Autodesk Inventor part; units mm, degrees
ref_plane "YZ Plane" through (0, 0, 0) normal (1, 0, 0) x (0, 1, 0)
ref_plane "XZ Plane" through (0, 0, 0) normal (0, 1, 0) x (-1, 0, 0)
ref_plane "XY Plane" through (0, 0, 0) normal (0, 0, 1) x (1, 0, 0)
sketch "Sketch1" plane through (0, 0, 0) normal (0, 1, 0) x (-1, 0, 0)
  line L0 (0, 0) -> (12.5, 0)
  line L1 (12.5, 0) -> (12.5, -22.9)
  line L2 (12.5, -22.9) -> (0, -22.9)
  line L3 (0, -22.9) -> (0, 0)
  line L4 (12.5, 0) -> (13, 0)
  line L5 (0, -22.9) -> (-0.5, -22.9)
  line L6 (13, 0) -> (13, 4.65)
  line L7 (-0.5, -22.9) -> (-0.5, -27.55)
  line L8 (13, 4.65) -> (-0.5, 4.65)
  line L9 (-0.5, 4.65) -> (-0.5, -27.55)
  line L10 (-0.5, -27.55) -> (13, -27.55)
  line L11 (13, -27.55) -> (13, 4.65)
  line L12 (6.25, 0) -> (6.25, 2.45)
  line L13 (6.25, -22.9) -> (6.25, -25.35)
  circle A0 centre (6.25, 2.45) radius 0.75
  circle A1 centre (6.25, -25.35) radius 0.75
  dimension "d0" = 12.5
  dimension "d1" = 22.9
  dimension "d2" = 0.5
  dimension "d3" = 0.5
  dimension "d4" = 4.65
  dimension "d5" = 4.65
  dimension "d6" = 2.45
  dimension "d7" = 2.45
  dimension "d8" = 1.5
  dimension "d9" = 1.5
extrude "Extrusion1" add sketch "Sketch1" along normal blind 17.3 contours A0 | L3 L5 L9 L8 L6 L4 L0 | A1 | L2 L1 L4 L11 L10 L7 L5
extrude "Extrusion2" add sketch "Sketch1" against normal blind 1 contours A0 | L3 L5 L9 L8 L6 L4 L0 | L0 L1 L2 L3 | A1 | L2 L1 L4 L11 L10 L7 L5
sketch "Sketch2" plane through (0, -1, 0) normal (0, -1, 0) x (1, 0, 0)
  line L0 (0.5, 4.65) -> (0.5, -27.55)
  line L1 (-12.5, -22.9) -> (0, -22.9)
  line L2 (-13, -27.55) -> (-13, 4.65)
  line L3 (-13, 4.65) -> (-13, 0)
  line L4 (-13, 0) -> (-6.3, 0)
  line L5 (0, 0) -> (-12.5, 0)
  line L6 (-6.3, 0) -> (-6.3, -5.6)
  circle A0 centre (-6.3, -5.6) radius 3.025
  dimension "d20" = 4.65
  dimension "d21" = 6.7
  dimension "d22" = 5.6
  dimension "d23" = 6.05
extrude "Extrusion3" add sketch "Sketch2" along normal blind 4.7
sketch "Sketch3" plane through (-6.3, -5.7, -5.6) normal (0, -1, 0) x (1, 0, 0)
  line L0 (0, 0) -> (1.385, 0)
  line L1 (0, 0) -> (0, 1.385)
  line L2 (1.385, 0) -> (1.385, 0.32)
  line L3 (0, 1.385) -> (-0.32, 1.385)
  line L4 (-0.32, 1.385) -> (0.32, 1.385)
  line L5 (0.32, 1.385) -> (0.32, -1.385)
  line L6 (0.32, -1.385) -> (-0.32, -1.385)
  line L7 (-0.32, -1.385) -> (-0.32, 1.385)
  line L8 (1.385, 0.32) -> (-1.385, 0.32)
  line L9 (-1.385, 0.32) -> (-1.385, -0.32)
  line L10 (-1.385, -0.32) -> (1.385, -0.32)
  line L11 (1.385, -0.32) -> (1.385, 0.32)
  point P0 (6.3, 5.6)
  point P1 (-0.32, 0.32)
  point P2 (-0.32, -0.32)
  point P3 (0.32, -0.32)
  point P4 (0.32, 0.32)
  dimension "d24" = 1.385
  dimension "d25" = 1.385
  dimension "d26" = 0.32
  dimension "d27" = 0.32
  dimension "d28" = 0.64
  dimension "d30" = 2.77
  dimension "d31" = 0.64
  dimension "d32" = 2.77
extrude "Extrusion4" [suppressed]
sketch "Sketch7" plane through (-13, 17.3, 4.65) normal (0, 0, 1) x (1, 0, 0)
  line L0 (0, -18.3) -> (13.5, -18.3)
  line L1 (6.75, -18.3) -> (6.75, -17.3)
  line L2 (6.75, -17.3) -> (2.25, -17.3)
  line L3 (0.5, -17.3) -> (13, -17.3)
  line L4 (2.25, -17.3) -> (11.25, -17.3)
  line L5 (11.25, -17.3) -> (11.25, -12.8)
  line L6 (11.25, -12.8) -> (2.25, -12.8)
  line L7 (2.25, -12.8) -> (2.25, -17.3)
  dimension "d47" = 1
  dimension "d48" = 4.5
  dimension "d49" = 4.5
  dimension "d50" = 9
extrude "Extrusion7" cut sketch "Sketch7" against normal up to next
sketch "Sketch8" plane through (-6.3, -5.7, -5.6) normal (0, -1, 0) x (1, 0, 0)
  line L0 (0, 0) -> (0, 1.7)
  line L1 (0, 1.7) -> (0.37, 1.7)
  line L2 (0.37, 1.7) -> (0.37, -1.7)
  line L3 (0.37, -1.7) -> (-0.37, -1.7)
  line L4 (-0.37, -1.7) -> (-0.37, 1.7)
  line L5 (-0.37, 1.7) -> (0, 1.7)
  line L6 (0, 0) -> (1.2021, -1.2021)
  line L7 (1.2021, -1.2021) -> (0.9405, -1.4637)
  line L8 (0.9405, -1.4637) -> (-1.4637, 0.9405)
  line L9 (-1.4637, 0.9405) -> (-0.9405, 1.4637)
  line L10 (-0.9405, 1.4637) -> (1.4637, -0.9405)
  line L11 (1.4637, -0.9405) -> (1.2021, -1.2021)
  point P0 (6.3, 5.6)
  dimension "d53" = 1.7
  dimension "d54" = 0.37
  dimension "d55" = 3.4
  dimension "d56" = 0.74
  dimension "d57" = 3.4
  dimension "d60" = 1.7
  dimension "d61" = 0.37
  dimension "d62" = 3.4
  dimension "d63" = 0.74
  dimension "d64" = 3.4
extrude "Extrusion8" cut sketch "Sketch8" against normal blind 3 contours L6 L2 L8 L4 L10 L0 | L0 L10 L2 L6 | L6 L7 L8 L2 | L2 L10 L11 L6 | L4 L8 L9 L10
properties part number "Servo Top Mount"
Verification items for the finished model (mm, model axes). A direction names the side the tool comes from. Round coordinates to 2 decimals unless told otherwise and drop trailing zeros. Order: outer loops, then holes, each group sorted by start corner. A loop starts at its lowest first (then second) coordinate and runs counter-clockwise, first axis right, second up.
1. Section check B-B on x = -5.75. Record the cut outline in (y, z).
Final values:
outline: (-5.7, -8.57) - (-1, -8.57) - (-1, -27.55) - (17.3, -27.55) - (17.3, -22.9) - (0, -22.9) - (0, 4.65) - (-1, 4.65) - (-1, -2.63) - (-5.7, -2.63) - (-5.7, -5.63) - (-2.7, -5.63) - (-2.7, -6.67) - (-5.7, -6.67) - close; (4.5, 0) - (17.3, 0) - (17.3, 4.65) - (4.5, 4.65) - close
2. Section check A-A on y = 8. Record the cut outline in (x, z), then the cut area to 3 significant figures.
Final values:
outline: (-13, -27.55) - (0.5, -27.55) - (0.5, 4.65) - (-13, 4.65) - close; hole (-12.5, -22.9) - (0, -22.9) - (0, 0) - (-12.5, 0) - close
area: 148 mm2
3. Access from +Z, -Z, +X, -X, +Y, -Y to the whole of each face (thin tool, end or side, straight path). Record for faces 5 (the flat face through (-6, 8, 4.65)), 6 (the flat face through (-6, 9, -22.9)), 7 (the flat face through (-6.545, -4.221, -5.878)), 8 (the flat face through (0.5, 8, -11)), 9 (the flat face through (-6, 0, -9)).
Final values:
face 5: +Z, +X, -X, +Y, -Y
face 6: +Y
face 7: -Y
face 8: +Z, -Z, +X, +Y, -Y
face 9: none
4. Thickness scan on L1, parallel to Z at x = -4.75, y = 16.75; L2, parallel to X at y = 6.75, z = -10; L3, parallel to Y at x = -10.5, z = 2. Record the ranges inside material, lowest first.
Final values:
L1: z = -27.55 to -22.9, 0 to 4.65
L2: x = -13 to -12.5, 0 to 0.5
L3: y = -1 to 0, 4.5 to 17.3
5. Go/stop test with flat-tipped pins: P1, Ø4, axis at x = -4, z = -5, coming from the +Y side; P2, Ø1, axis at x = -8.5, z = -19, coming from the -Y side. Record where each tip stops, or that it passes through.
Final values:
P1: stops at y = 0
P2: stops at y = -1
6. Section check C-C on z = -20.5. Record the cut outline in (x, y).
Final values:
outline: (-13, -1) - (0.5, -1) - (0.5, 17.3) - (0, 17.3) - (0, 0) - (-12.5, 0) - (-12.5, 17.3) - (-13, 17.3) - close
7. Release check for a two-part mould opening along Y. For faces 1 (the flat face through (-6, -2.7, -6)), 2 (the flat face through (-13, 8, -12)), 3 (the flat face through (-1.75, 2, 2)), 4 (the flat face through (-6, 4.5, 2)) record: +Y half, -Y half, draft (parallel to the pull), parting line (faces both ways), or undercut.
Final values:
face 1: -Y half
face 2: draft
face 3: undercut
face 4: undercut
8. Section check D-D on y = 2.75. Record the cut outline in (x, z), then the cut area to 3 significant figures.
Final values:
outline: (-13, -27.55) - (0.5, -27.55) - (0.5, 4.65) - (-1.75, 4.65) - (-1.75, 0) - (0, 0) - (0, -22.9) - (-12.5, -22.9) - (-12.5, 0) - (-10.75, 0) - (-10.75, 4.65) - (-13, 4.65) - close
area: 107 mm2
